```python
from build123d import *

# Parameters (mm, degrees)
F0_R     = 3.4
F1_DEPTH = 1.5
F0_R_2   = 1.5
F2_DEPTH = 5
F3_DEPTH = 2
F4_SIZE  = 1
F5_R     = 0.99999
F6_R     = 0.5


# Not quite as in the source:
# - a fillet or chamfer is up to 0.001 mm smaller than in the source, because OpenCascade refuses the exact size


with BuildPart() as f1:
    # F0 (on Top) → F1 (new body)
    with BuildSketch(Plane.XY):
        Polygon((4.5, -2.5980762114), (4.5, 2.5980762114), (0, 5.1961524227), (-4.5, 2.5980762114), (-4.5, -2.5980762114), (0, -5.1961524227), align=None)
        Circle(F0_R, mode=Mode.SUBTRACT)
    extrude(amount=F1_DEPTH)

    # F0 (on Top) → F2 (join)
    with BuildSketch(Plane.XY):
        Circle(F0_R)
        Circle(F0_R_2, mode=Mode.SUBTRACT)
        Circle(F0_R_2)
    extrude(amount=F2_DEPTH)

    # F0 (on Top) → F3 (cut)
    with BuildSketch(Plane.XY):
        Circle(F0_R_2)
    extrude(amount=F3_DEPTH, mode=Mode.SUBTRACT)

    # F4
    f4_edges = [f1.edges().sort_by_distance(p)[0] for p in [
        (4.5, 0, 0),
        (2.25, -3.897114, 0),
        (2.25, 3.897114, 0),
        (-2.25, -3.897114, 0),
        (-2.25, 3.897114, 0),
        (-4.5, 0, 0),
        (-1.5, 0, 0),
    ]]
    chamfer(f4_edges, length=F4_SIZE)

    # F5 (radius 1 in the source; OpenCascade refuses exactly that, so slightly less here)
    f5_edges = [f1.edges().sort_by_distance(p)[0] for p in [
        (-1.5, 0, 2),
    ]]
    fillet(f5_edges, radius=F5_R)

    # F6
    f6_edges = [f1.edges().sort_by_distance(p)[0] for p in [
        (-3.4, 0, 5),
    ]]
    fillet(f6_edges, radius=F6_R)


solid = f1.part
```
The model under review builds one solid part; all positions refer to its coordinate system, in mm. A direction names the side the tool comes from. Give positions to 0.01 mm unless a question says otherwise; leave off trailing zeros. Write each loop counter-clockwise with the first axis right and the second up, starting at its lowest first coordinate (ties: lowest second). Pieces come first, ordered by that corner, then holes.
(1) The part is to be moulded in two halves that separate along X. For faces 3 (the flat face through (-2.28, -3.88, 1.25)), 4 (the flat face through (0, 0, 2)), 5 (the flat face through (-2, -3, 1.5)), say which applies: released by +X, released by -X, zero draft, split by the parting line, or undercut.
(2) Consider section A-A, the plane z = 2.5. Give the boundary of the cut face in (x, y), and give its area (3 significant figures).
(3) Tool access review of faces 1 (the flat face through (-4, 0, 0.5)), 2 (the cylindrical face through (-0.74, -3.32, 2.98)): name each direction out of +Z, -Z, +X, -X, +Y, -Y from which nothing blocks a thin tool from reaching the whole face with its end or side.
(4) For P1, Ø3, axis at x = -3.5, z = 1, coming from the +Y side, flat-tipped, find the tip position at first contact; note if it passes through.
(5) To check wall thickness, follow L1, parallel to X at y = 0, z = 1.05; L2, parallel to Y at x = -0.25, z = 0.95; L3, parallel to Y at x = -1.75, z = 0.55. State the ranges of each line that lie inside material, in increasing order.
Returned:
1. face 3: released by -X
1. face 4: undercut
1. face 5: zero draft
2. outline: circle Ø6.8 at (0, 0)
2. area: 36.3 mm2
3. face 1: -Z, -X, +Y, -Y
3. face 2: +Z
4. P1: stops at y = 4.04
5. L1: x = -4.5 to -1.5, 1.5 to 4.5
5. L2: y = -4.99 to -1.53, 1.53 to 4.99
5. L3: y = -3.67 to -0.86, 0.86 to 3.67
